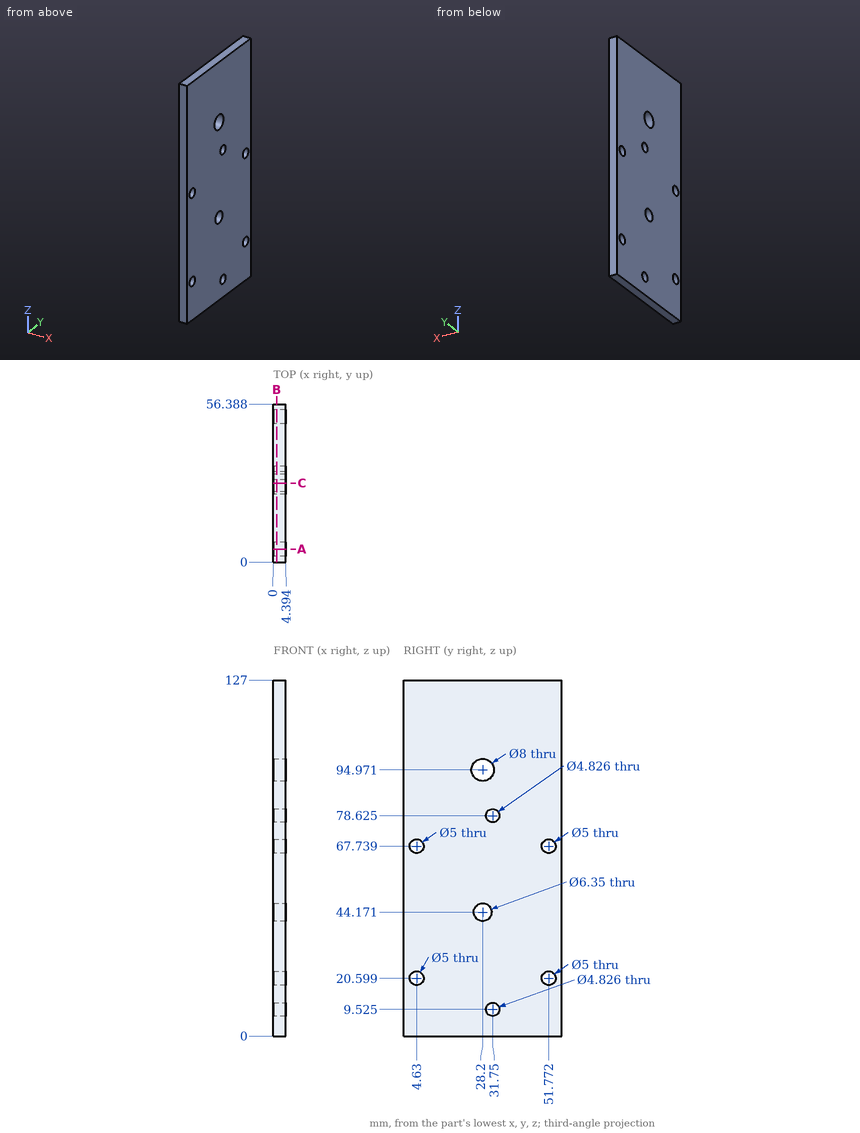
Print and shaded views of the part. All mm, measured from the part's lowest x, y and z. Coordinates: 2 decimals unless noted, no trailing zeros. Order: outer loops, then holes, each group sorted by start corner. A loop starts at its lowest first (then second) coordinate and runs counter-clockwise, first axis right, second up. Notation, with made-up numbers: (8.25, 38.5) - (63.25, 38.5) arc R7 cw to (63.25, 44.5) - close; hole circle Ø6 at (85, 48.25). An arc over 180 degrees is marked (long way). Return JSON: item names as keys, results as strings. Group by question number.
Item 1: Cut at C-C (y = 28.2). List the corners of the cut face in (x, z) (1 decimal), plus the area to 3 significant figures.
Item 2: Pin check, flat tip, straight feed: pin 1 (4 mm diameter, centred on y = 4.63, z = 20.6, fed in from -X). Stop position of the tip, or through.
Item 3: Drill centre lines: probe 1 along Z at (x, y) = (2.5, 4.63); probe 2 along Z at (x, y) = (3.15, 28.2) (1 decimal); probe 3 along Y at (x, z) = (3.2, 97). Where is each one in solid material? Low to high. Write a range as from..to.
Item 4: Cut at A-A (y = 4.63). List the corners of the cut face in (x, z) (1 decimal).
Item 5: Cut at B-B (x = 1.2). State how many separate pieces and enclosed holes the cut face has, plus the area to 3 significant figures.
Check values:
{
 "1": {"outline": "(0, 0) - (4.4, 0) - (4.4, 41) - (0, 41) - close; (0, 47.3) - (4.4, 47.3) - (4.4, 91) - (0, 91) - close; (0, 99) - (4.4, 99) - (4.4, 127) - (0, 127) - close", "area": "495 mm2"},
 "2": {"pin 1": "passes through"},
 "3": {"probe 1": "z = 0..18.1, 23.1..65.24, 70.24..127", "probe 2": "z = 0..41, 47.3..91, 99..127", "probe 3": "y = 0..24.75, 31.65..56.39"},
 "4": {"outline": "(0, 0) - (4.4, 0) - (4.4, 18.1) - (0, 18.1) - close; (0, 23.1) - (4.4, 23.1) - (4.4, 65.2) - (0, 65.2) - close; (0, 70.2) - (4.4, 70.2) - (4.4, 127) - (0, 127) - close"},
 "5": {"separate pieces": "1", "enclosed holes": "8", "area": "6,960 mm2"}
}
